from build123d import *

# Parameters (mm, degrees)
SKETCH_1_W          = 100
SKETCH_1_H          = 70
EXTRUDE_1_DEPTH     = 5
SKETCH_2_W          = 10
SKETCH_2_H          = 12
SKETCH_2_W_2        = 5
CUT_EXTRUDE_1_DEPTH = 10
SKETCH_3_R          = 1.5
CUT_EXTRUDE_2_DEPTH = 5


with BuildPart() as part:
    # 스케치1 → 보스-돌출1 (new body)
    with BuildSketch(Plane(origin=(0, 0, 0), x_dir=(1, 0, 0), z_dir=(0, 1, 0))):
        with Locations((50, 35)):
            Rectangle(SKETCH_1_W, SKETCH_1_H)
    extrude(amount=EXTRUDE_1_DEPTH)

    # 스케치2 → 컷-돌출1 (cut)
    with BuildSketch(Plane(origin=(0, 5, 0), x_dir=(1, 0, 0), z_dir=(0, 1, 0))):
        with Locations((58.07, 47)):
            Rectangle(SKETCH_2_W, SKETCH_2_H)
        with Locations((58.07, 23)):
            Rectangle(SKETCH_2_W, SKETCH_2_H)
        with Locations((81, 47)):
            Rectangle(SKETCH_2_W_2, SKETCH_2_H)
        with Locations((81, 23)):
            Rectangle(SKETCH_2_W_2, SKETCH_2_H)
        with Locations((11.07, 47)):
            Rectangle(SKETCH_2_W_2, SKETCH_2_H)
        with Locations((11.07, 23)):
            Rectangle(SKETCH_2_W_2, SKETCH_2_H)
    extrude(amount=-CUT_EXTRUDE_1_DEPTH, mode=Mode.SUBTRACT)

    # 스케치3 → 컷-돌출2 (cut)
    with BuildSketch(Plane(origin=(0, 5, 0), x_dir=(1, 0, 0), z_dir=(0, 1, 0))):
        with Locations((8.57, 51.5)):
            Circle(SKETCH_3_R)
        with Locations((13.57, 51.5)):
            Circle(SKETCH_3_R)
        with Locations((8.57, 42.5)):
            Circle(SKETCH_3_R)
        with Locations((13.57, 42.5)):
            Circle(SKETCH_3_R)
        with Locations((8.57, 27.5)):
            Circle(SKETCH_3_R)
        with Locations((13.57, 27.5)):
            Circle(SKETCH_3_R)
        with Locations((13.57, 18.5)):
            Circle(SKETCH_3_R)
        with Locations((8.57, 18.5)):
            Circle(SKETCH_3_R)
        with Locations((63.07, 18.5)):
            Circle(SKETCH_3_R)
        with Locations((53.07, 18.5)):
            Circle(SKETCH_3_R)
        with Locations((53.07, 27.5)):
            Circle(SKETCH_3_R)
        with Locations((63.07, 27.5)):
            Circle(SKETCH_3_R)
        with Locations((78.5, 27.5)):
            Circle(SKETCH_3_R)
        with Locations((83.5, 27.5)):
            Circle(SKETCH_3_R)
        with Locations((78.5, 18.5)):
            Circle(SKETCH_3_R)
        with Locations((83.5, 18.5)):
            Circle(SKETCH_3_R)
        with Locations((78.5, 42.5)):
            Circle(SKETCH_3_R)
        with Locations((83.5, 42.5)):
            Circle(SKETCH_3_R)
        with Locations((78.5, 51.5)):
            Circle(SKETCH_3_R)
        with Locations((83.5, 51.5)):
            Circle(SKETCH_3_R)
        with Locations((63.07, 51.5)):
            Circle(SKETCH_3_R)
        with Locations((53.07, 51.5)):
            Circle(SKETCH_3_R)
        with Locations((53.07, 42.5)):
            Circle(SKETCH_3_R)
        with Locations((63.07, 42.5)):
            Circle(SKETCH_3_R)
    extrude(amount=-CUT_EXTRUDE_2_DEPTH, mode=Mode.SUBTRACT)


solid = part.part
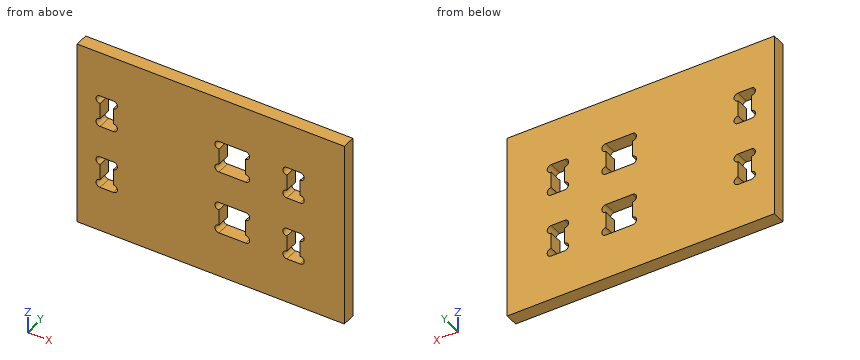
Build history of the part. All positions in model axes, mm. Round coordinates to 2 decimals unless told otherwise and drop trailing zeros. Write each loop counter-clockwise with the first axis right and the second up, starting at its lowest first coordinate (ties: lowest second). Pieces come first, ordered by that corner, then holes. Notation, with made-up numbers: (8.25, -1) - (17.25, -1) arc R31 ccw to (17.25, 23) - close; hole circle Ø9 at (43.25, -34). An arc over 180 degrees is marked (long way). Use CSV: the item, a comma, the result in double quotes.
(1) Band-saw the part on A-A (z = -42.5). Write the cut outline in (x, y), plus the area to 3 significant figures.
Response:
outline,"(0, 0) - (7.07, 0) - (7.07, 5) - (0, 5) - close; (15.07, 0) - (51.57, 0) - (51.57, 5) - (15.07, 5) - close; (64.57, 0) - (77, 0) - (77, 5) - (64.57, 5) - close; (85, 0) - (100, 0) - (100, 5) - (85, 5) - close"
area,"355 mm²"
(2) Band-saw the part on B-B (y = 1.45). Give the number of separate pieces and of enclosed holes in the cut face, plus the area to 3 significant figures.
Response:
separate pieces,"1"
enclosed holes,"6"
area,"6,440 mm²"
(3) Wall check: line 1 (Z direction, x = 8.5, y = 3.55); line 2 (X direction, y = 0.6, z = -46); line 3 (Z direction, x = 12.5, y = 3.7). Give the ranges that are in metal, low to high.
Response:
line 1,"-70 to -53, -50 to -44, -41 to -29, -26 to -20, -17 to 0"
line 2,"0 to 8.57, 13.57 to 53.07, 63.07 to 78.5, 83.5 to 100"
line 3,"-70 to -53, -41 to -29, -17 to 0"
